Here's how the part is built. I have some questions about the finished solid (model axes, mm). A direction names the side the tool comes from. Coordinates: 2 decimals unless noted, no trailing zeros. Write each loop counter-clockwise with the first axis right and the second up, starting at its lowest first coordinate (ties: lowest second). Pieces come first, ordered by that corner, then holes.
Item 1: For faces 4 (the face through (-38, 51, 30)), 5 (the face through (-1, 9, 53)), 6 (the face through (-40, 76, 6)), which set-ups out of +Z, -Z, +X, -X, +Y, -Y let a thin tool reach every point of the face, with its end or its side?
Item 2: If we section it at A-A (z = 66): Please give me the cut outline in (x, y).
Item 3: We'd pull the mould along Y, two halves only. Please class faces 1 (the face through (59.957, 1.112, 25.349)), 2 (the face through (-1, -7, 45)), 3 (the face through (-65.45, 63.66, 18.12)): +Y half, -Y half, draft (parallel to the pull), parting line (faces both ways), or undercut.
Item 4: If I drill on line 1 (X direction, y = -2, z = 66); line 2 (Y direction, x = 7, z = 25); line 3 (Z direction, x = 37, y = 122), over which ranges is the centre line in solid material (lowest first)?
Item 5: If we section it at B-B (z = 26): Please give me the cut outline in (x, y).
Item 6: I'm going to push flat-ended pins straight in: pin 1 Ø11.5 at (x, z) = (55, 26) entering from -Y; pin 2 Ø1 at (y, z) = (107, 20) entering from -X; pin 3 Ø3.5 at (y, z) = (112, 5) entering from -X. Where does each tip first touch, or does it pass through?
Item 7: If we section it at D-D (y = 63): Please give me the cut outline in (x, z).
Item 8: If we section it at C-C (x = -55): Please give me the cut outline in (y, z).
from build123d import *

# Parameters (mm, degrees)
SKETCH1_W               = 133.951426206
SKETCH1_H               = 18
BOSS_EXTRUDE1_DEPTH     = 96
BOSS_EXTRUDE2_DEPTH     = 12
SKETCH1_4_R             = 20
SKETCH1_4_R_2           = 10
BOSS_EXTRUDE3_DEPTH     = 30
SKETCH1_5_R             = 25
SKETCH1_5_R_2           = 15
BOSS_EXTRUDE4_DEPTH     = 35
CUT_EXTRUDE1_DEPTH      = 219.192540162
CUT_EXTRUDE1_DEPTH_BACK = 140
SKETCH2_W               = 60
SKETCH2_H               = 2
SKETCH4_R               = 5
CUT_EXTRUDE3_DEPTH      = 35
SKETCH5_R               = 5
CUT_EXTRUDE4_DEPTH      = 35


with BuildPart() as part:
    # Sketch1 → Boss-Extrude1 (new body)
    with BuildSketch(Plane.XY):
        Rectangle(SKETCH1_W, SKETCH1_H)
    extrude(amount=BOSS_EXTRUDE1_DEPTH)

    # Sketch1_3 → Boss-Extrude2 (add)
    with BuildSketch(Plane.XY):
        with BuildLine():
            Line((-66.975713103, 9), (66.975713103, 9))
            Line((66.975713103, 9), (41.975713103, 118))
            ThreePointArc((41.975713103, 118), (16.975713103, 93), (-8.024286897, 118))
            Line((-8.024286897, 118), (-8.024286897, 101))
            ThreePointArc((-8.024286897, 101), (-15.346617368, 83.32233047), (-33.024286897, 76))
            Line((-33.024286897, 76), (-46.975713103, 76))
            ThreePointArc((-46.975713103, 76), (-32.833577479, 70.142135624), (-26.975713103, 56))
            ThreePointArc((-26.975713103, 56), (-46.975713103, 36), (-66.975713103, 56))
            Line((-66.975713103, 56), (-66.975713103, 9))
        make_face()
    extrude(amount=BOSS_EXTRUDE2_DEPTH)

    # Sketch1_4 → Boss-Extrude3 (add)
    with BuildSketch(Plane.XY):
        with Locations(Location((-46.975713103, 56, 0), (0, 0, 180))):
            Circle(SKETCH1_4_R)
        with Locations((-46.975713103, 56)):
            Circle(SKETCH1_4_R_2, mode=Mode.SUBTRACT)
    extrude(amount=BOSS_EXTRUDE3_DEPTH)

    # Sketch1_5 → Boss-Extrude4 (add)
    with BuildSketch(Plane.XY):
        with Locations((16.975713103, 118)):
            Circle(SKETCH1_5_R)
        with Locations((16.975713103, 118)):
            Circle(SKETCH1_5_R_2, mode=Mode.SUBTRACT)
    extrude(amount=BOSS_EXTRUDE4_DEPTH)

    # Sketch2 → Cut-Extrude1 (cut, two sides: drawn at the far end of the back side and taken through both)
    with BuildSketch(Plane(origin=(66.975713103, 0, 0), x_dir=(0, 0, -1), z_dir=(1, 0, 0)).offset(-CUT_EXTRUDE1_DEPTH_BACK)):
        with Locations((-45, -8)):
            Rectangle(SKETCH2_W, SKETCH2_H)
    extrude(amount=CUT_EXTRUDE1_DEPTH + CUT_EXTRUDE1_DEPTH_BACK, mode=Mode.SUBTRACT)

    # Sketch4 → Cut-Extrude3 (cut)
    with BuildSketch(Plane(origin=(0, 9, 0), x_dir=(1, 0, 0), z_dir=(0, 1, 0))):
        with Locations(Location((55, -26, 0), (0, 0, 270))):
            Circle(SKETCH4_R)
        with Locations(Location((55, -66, 0), (0, 0, 270))):
            Circle(SKETCH4_R)
        with Locations(Location((-55, -66, 0), (0, 0, 270))):
            Circle(SKETCH4_R)
    extrude(amount=-CUT_EXTRUDE3_DEPTH, mode=Mode.SUBTRACT)

    # Sketch5 → Cut-Extrude4 (cut)
    with BuildSketch(Plane(origin=(0, 9, 0), x_dir=(1, 0, 0), z_dir=(0, 1, 0))):
        with Locations(Location((-55, -26, 0), (0, 0, 270))):
            Circle(SKETCH5_R)
    extrude(amount=-CUT_EXTRUDE4_DEPTH, mode=Mode.SUBTRACT)


solid = part.part
Answer list:
1. face 4: +Z, +X, -X, +Y
1. face 5: +Z, +X, -X
1. face 6: +Z, -Z, -X, +Y
2. outline: (-66.98, -7) - (-60, -7) - (-60, 9) - (-66.98, 9) - close; (-50, -7) - (50, -7) - (50, 9) - (-50, 9) - close; (60, -7) - (66.98, -7) - (66.98, 9) - (60, 9) - close
3. face 1: draft
3. face 2: -Y half
3. face 3: undercut
4. line 1: x = -66.98 to -60, -50 to 50, 60 to 66.98
4. line 2: y = -7 to 9, 95.08 to 106.8, 129.2 to 140.92
4. line 3: z = 0 to 35
5. outline: (-66.98, -7) - (-60, -7) - (-60, 9) - (-66.98, 9) - close; circle Ø40 at (-46.98, 56); (-50, -7) - (50, -7) - (50, 9) - (-50, 9) - close; circle Ø50 at (16.98, 118); (60, -7) - (66.98, -7) - (66.98, 9) - (60, 9) - close; hole circle Ø20 at (-46.98, 56); hole circle Ø30 at (16.98, 118)
6. pin 1: stops at y = -7
6. pin 2: stops at x = -5.71
6. pin 3: stops at x = -8.02
7. outline: (-65.71, 0) - (-54.12, 0) - (-54.12, 30) - (-65.71, 30) - close; (-39.83, 0) - (54.59, 0) - (54.59, 12) - (-28.24, 12) - (-28.24, 30) - (-39.83, 30) - close
8. outline: (-9, 0) - (50.03, 0) - (50.03, 30) - (37.68, 30) - (37.68, 12) - (9, 12) - (9, 21) - (-7, 21) - (-7, 15) - (-9, 15) - close; (-9, 75) - (-7, 75) - (-7, 71) - (9, 71) - (9, 96) - (-9, 96) - close; (-7, 31) - (9, 31) - (9, 61) - (-7, 61) - close; (61.97, 0) - (74.32, 0) - (74.32, 30) - (61.97, 30) - close
